Can you work these out from the drawing? Everything is in mm from the part's minimum corner. A direction names the side the tool comes from. Coordinates: 2 decimals unless noted, no trailing zeros. Loops run counter-clockwise (first coordinate to the right, second up) from the corner with the lowest first, then second, coordinate; pieces in that order, holes last. Notation, with made-up numbers: (71.25, -28) - (104.25, -28) arc R23 cw to (104.25, 4) - close; hole circle Ø3 at (41.25, 68.25). An arc over 180 degrees is marked (long way). Use CSV: the item, a comma, the result in double quotes.
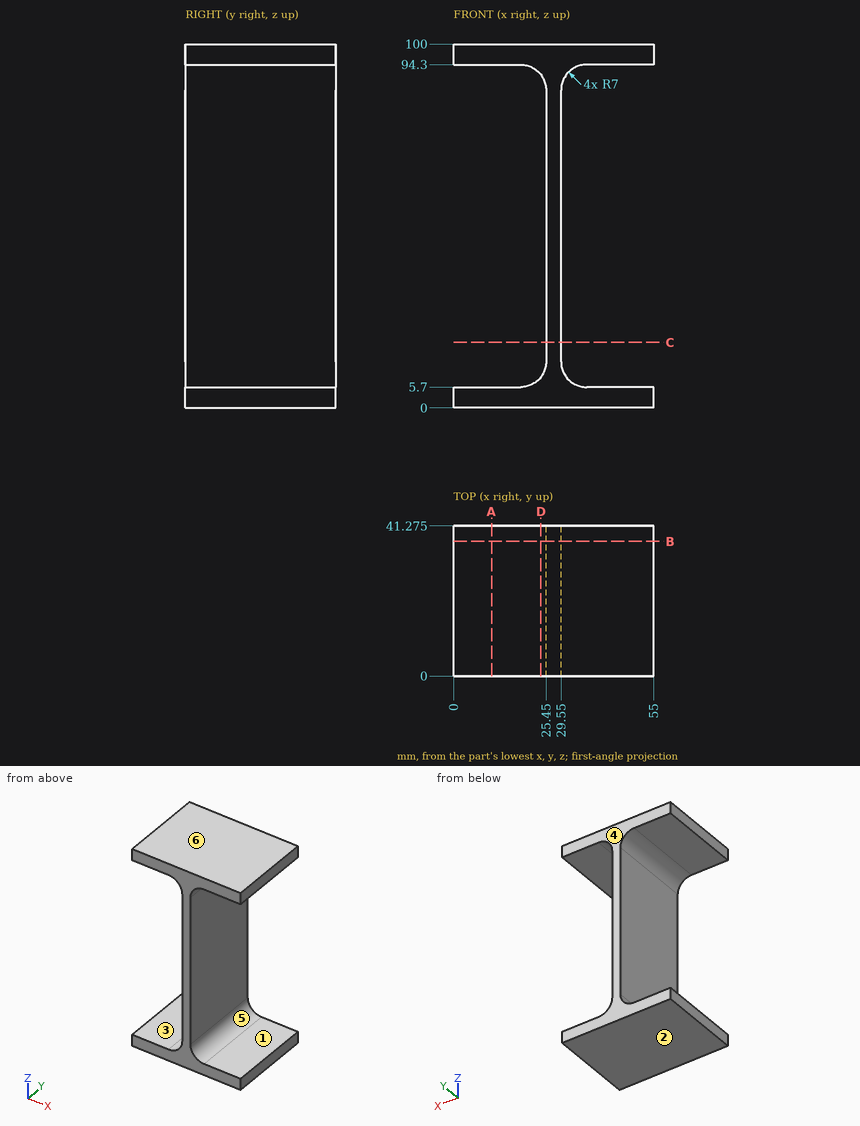
(1) Which directions (+Z, -Z, +X, -X, +Y, -Y) give clear straight access to the entire face, cutting with the end or side of a thin tool? Please do the marked faces 1, 2 and 3.
Computed:
face 1,"+X, +Y, -Y"
face 2,"-Z, +X, -X, +Y, -Y"
face 3,"-X, +Y, -Y"
(2) Suppose I cut it at C-C (z = 18). Write out the boundary of the cut face in (x, y) (3 decimals).
Computed:
outline,"(25.45, 0) - (29.55, 0) - (29.55, 41.275) - (25.45, 41.275) - close"
(3) Suppose I cut it at A-A (x = 10.5). Write out the boundary of the cut face in (y, z) (3 decimals), plus the area to 3 significant figures.
Computed:
outline,"(0, 0) - (41.275, 0) - (41.275, 5.7) - (0, 5.7) - close; (0, 94.3) - (41.275, 94.3) - (41.275, 100) - (0, 100) - close"
area,"471 mm²"
(4) Will this pin go through, and if not, where does the flat tip stop? pin 1 (4 mm diameter, centred on y = 34.5, z = 39, fed in from +X).
Computed:
pin 1,"stops at x = 29.55"
(5) Please list where these lines run through material, in increasing order: line 1 (Z direction, x = 50.5, y = 4); line 2 (X direction, y = 33, z = 80); line 3 (Z direction, x = 24, y = 13).
Computed:
line 1,"z = 0 to 5.7, 94.3 to 100"
line 2,"x = 25.45 to 29.55"
line 3,"z = 0 to 8.43, 91.57 to 100"
(6) Suppose I cut it at D-D (x = 24). Write out the boundary of the cut face in (y, z) (3 decimals).
Computed:
outline,"(0, 0) - (41.275, 0) - (41.275, 8.434) - (0, 8.434) - close; (0, 91.566) - (41.275, 91.566) - (41.275, 100) - (0, 100) - close"
(7) Thinking about a two-plate mould opening in Z: for the marked faces 4, 5 and 6, which applies, +Z half, -Z half, draft (parallel to the pull), parting line (faces both ways), or undercut?
Computed:
face 4,"draft"
face 5,"undercut"
face 6,"+Z half"
(8) Suppose I cut it at B-B (y = 37). Write out the boundary of the cut face in (x, z).
Computed:
outline,"(0, 0) - (55, 0) - (55, 5.7) - (36.55, 5.7) arc R7 cw to (29.55, 12.7) - (29.55, 87.3) arc R7 cw to (36.55, 94.3) - (55, 94.3) - (55, 100) - (0, 100) - (0, 94.3) - (18.45, 94.3) arc R7 cw to (25.45, 87.3) - (25.45, 12.7) arc R7 cw to (18.45, 5.7) - (0, 5.7) - close"
